from build123d import *

# Parameters (mm, degrees)
SKETCH_W        = 79
SKETCH_H        = 25
PAD_DEPTH       = 2
SKETCH001_W     = 21
SKETCH001_H     = 25
PAD001_DEPTH    = 4.85
SKETCH002_R     = 1.5
POCKET_DEPTH    = 25.001
SKETCH003_W     = 21
SKETCH003_H     = 12
POCKET001_DEPTH = 10
PAD002_DEPTH    = 6.85
SKETCH005_W     = 9
SKETCH005_H     = 38.5
PAD003_DEPTH    = 18.15
SKETCH006_R     = 1.5
POCKET002_DEPTH = 10
SKETCH007_R     = 1.5
POCKET003_DEPTH = 22
FILLET_R        = 4.5
FILLET001_R     = 3


with BuildPart() as part:
    # Sketch → Pad (new body)
    with BuildSketch(Plane.XZ):
        Rectangle(SKETCH_W, SKETCH_H)
    extrude(amount=PAD_DEPTH)

    # Sketch001 (on Face5 of Pad) → Pad001 (join)
    with BuildSketch(Plane(origin=(0, 0, 0), x_dir=(1, 0, 0), z_dir=(0, 1, 0))):
        Rectangle(SKETCH001_W, SKETCH001_H)
    extrude(amount=PAD001_DEPTH)

    # Sketch002 (on Face5 of Pad001) → Pocket (cut, through all)
    with BuildSketch(Plane(origin=(0, 0, 12.5), x_dir=(-1, 0, 0), z_dir=(0, 0, 1))):
        with Locations((-5, -1.85)):
            Circle(SKETCH002_R)
        with Locations((5, -1.85)):
            Circle(SKETCH002_R)
    extrude(amount=-POCKET_DEPTH, mode=Mode.SUBTRACT)

    # Sketch003 (on Face11 of Pocket) → Pocket001 (cut)
    with BuildSketch(Plane(origin=(0, 4.85, 0), x_dir=(1, 0, 0), z_dir=(0, 1, 0))):
        with Locations((0, 6.5)):
            Rectangle(SKETCH003_W, SKETCH003_H)
    extrude(amount=-POCKET001_DEPTH, mode=Mode.SUBTRACT)

    # Sketch004 (on DatumPlane) → Pad002 (join)
    with BuildSketch(Plane(origin=(0, -2, 12.5), x_dir=(1, 0, 0), z_dir=(0, 0, -1))):
        Polygon((39.5, 0), (39.5, 7), (19.5, 7), (19.5, 38.5), (10.5, 38.5), (10.5, 0), align=None)
        Polygon((-19.5, 38.5), (-19.5, 7), (-39.5, 7), (-39.5, 0), (-10.5, 0), (-10.5, 38.5), align=None)
    extrude(amount=PAD002_DEPTH)

    # Sketch005 (on Face26 of Pad002) → Pad003 (join)
    with BuildSketch(Plane(origin=(0, 0, 5.65), x_dir=(1, 0, 0), z_dir=(0, 0, -1))):
        with Locations((-15, 21.25)):
            Rectangle(SKETCH005_W, SKETCH005_H)
        with Locations((15, 21.25)):
            Rectangle(SKETCH005_W, SKETCH005_H)
    extrude(amount=PAD003_DEPTH)

    # Sketch006 (on Face4 of Pad003) → Pocket002 (cut)
    with BuildSketch(Plane(origin=(0, 0, 0), x_dir=(1, 0, 0), z_dir=(0, 1, 0))):
        with Locations((24.5, -9.5)):
            Circle(SKETCH006_R)
        with Locations((34.5, -9.5)):
            Circle(SKETCH006_R)
        with Locations((-34.5, -9.5)):
            Circle(SKETCH006_R)
        with Locations((-24.5, -9.5)):
            Circle(SKETCH006_R)
    extrude(amount=-POCKET002_DEPTH, mode=Mode.SUBTRACT)

    # Sketch007 (on Face44 of Pocket002) → Pocket003 (cut)
    with BuildSketch(Plane.XZ.offset(40.5)):
        with Locations((15, -6.5)):
            Circle(SKETCH007_R)
        with Locations((15, 6.5)):
            Circle(SKETCH007_R)
        with Locations((-15, -6.5)):
            Circle(SKETCH007_R)
        with Locations((-15, 6.5)):
            Circle(SKETCH007_R)
    extrude(amount=-POCKET003_DEPTH, mode=Mode.SUBTRACT)

    # Fillet
    fillet_edges = [part.edges().sort_by_distance(p)[0] for p in [
        (-10.5, 0, 6),
        (10.5, 0, 6),
    ]]
    fillet(fillet_edges, radius=FILLET_R)

    # Fillet001
    fillet001_edges = [part.edges().sort_by_distance(p)[0] for p in [
        (10.5, 4.85, 6),
        (-10.5, 4.85, 6),
    ]]
    fillet(fillet001_edges, radius=FILLET001_R)


solid = part.part
Model file for the job. Use its own axes, mm. A direction names the side the tool comes from. Give positions to 0.01 mm unless a question says otherwise; leave off trailing zeros. Write each loop counter-clockwise with the first axis right and the second up, starting at its lowest first coordinate (ties: lowest second). Pieces come first, ordered by that corner, then holes. Notation, with made-up numbers: (38.25, -6.75) - (88.25, -6.75) arc R20 ccw to (88.25, 10.25) - close; hole circle Ø10 at (-20.5, -16). An arc over 180 degrees is marked (long way). Answer as CSV lines item,"result".
1. Band-saw the part on B-B (y = -3). Write the cut outline in (x, z).
Responses:
outline,"(-39.5, 5.65) - (-19.5, 5.65) - (-19.5, -12.5) - (-10.5, -12.5) - (-10.5, 12.5) - (-39.5, 12.5) - close; (10.5, -12.5) - (19.5, -12.5) - (19.5, 5.65) - (39.5, 5.65) - (39.5, 12.5) - (10.5, 12.5) - close; hole circle Ø3 at (-34.5, 9.5); hole circle Ø3 at (-24.5, 9.5); hole circle Ø3 at (24.5, 9.5); hole circle Ø3 at (34.5, 9.5)"
2. Band-saw the part on D-D (y = -12.5). Write the cut outline in (x, z).
Responses:
outline,"(-19.5, -12.5) - (-10.5, -12.5) - (-10.5, 12.5) - (-19.5, 12.5) - close; (10.5, -12.5) - (19.5, -12.5) - (19.5, 12.5) - (10.5, 12.5) - close"
3. Two-plate mould, pull along X, no slides. Class faces 1 (the face through (-16, -20, -12.5)), 2 (the face through (0, -2, 6)), 3 (the face through (-12.47, 0.78, 5.91)), 4 (the face through (39.5, -3, 6)): +X half, -X half, draft (parallel to the pull), parting line (faces both ways), or undercut.
Responses:
face 1,"draft"
face 2,"undercut"
face 3,"-X half"
face 4,"+X half"
4. Band-saw the part on C-C (z = -10). Write the cut outline in (x, y), and give its area (3 significant figures).
Responses:
outline,"(-39.5, -2) - (-19.5, -2) - (-19.5, -40.5) - (-10.5, -40.5) - (-10.5, 0) - (-39.5, 0) - close; (10.5, -40.5) - (19.5, -40.5) - (19.5, -2) - (39.5, -2) - (39.5, 0) - (10.5, 0) - close"
area,"809 mm2"
5. Band-saw the part on A-A (x = -5). Write the cut outline in (y, z), and give its area (4 significant figures).
Responses:
outline,"(-2, -0.5) - (0.35, -0.5) - (0.35, 12.5) - (-2, 12.5) - close; (3.35, -0.5) - (4.85, -0.5) - (4.85, 12.5) - (3.35, 12.5) - close"
area,"50.05 mm2"
6. Pin check, flat tips, straight feed: pin 1 (8 mm diameter, centred on x = -4.5, z = 5, fed in from -Y); pin 2 (2 mm diameter, centred on x = 29, y = -7, fed in from -Z); pin 3 (1.5 mm diameter, centred on y = -25.5, z = -4.5, fed in from -X). Stop position of each tip, or through.
Responses:
pin 1,"stops at y = -2"
pin 2,"stops at z = 5.65"
pin 3,"stops at x = -19.5"
7. Drill centre lines: L1, parallel to X at y = -3.25, z = 9.5; L2, parallel to Z at x = 15, y = -32; L3, parallel to Z at x = -15.5, y = -27.5. Where is each one in solid material? Low to high. Write a range as [from, to].
Responses:
L1,"x = [-39.5, -36], [-33, -26], [-23, -10.5], [10.5, 23], [26, 33], [36, 39.5]"
L2,"z = [-12.5, -8], [-5, 5], [8, 12.5]"
L3,"z = [-12.5, -7.91], [-5.09, 5.09], [7.91, 12.5]"
8. 3-axis set-ups, long thin cutter, end or side, ignore diameter. For faces 5 (the face through (-6.386, 2.425, 6.091)), 6 (the face through (13.5, -29.65, 6.57)), 7 (the face through (15, -40.5, 0)), 8 (the face through (30, -9, 9)), 9 (the face through (29, -6, 5.65)): which of +Z, -Z, +X, -X, +Y, -Y reach the whole face in a straight line?
Responses:
face 5,"+Z, -Z"
face 6,"-Y"
face 7,"+Z, -Z, +X, -X, -Y"
face 8,"+Z, -Z, +X, -Y"
face 9,"-Z, +X, -Y"
